Source: CAD feature listing. Evaluate the final solid. Frame: model axes, mm. Coordinates: 2 decimals unless noted, no trailing zeros. Loops run counter-clockwise (first coordinate to the right, second up) from the corner with the lowest first, then second, coordinate; pieces in that order, holes last. Notation, with made-up numbers: (34, 18.5) -> (63, 18.5) arc R21 ccw to (63, 37.5) -> close; hole circle Ø7 at (43, 70.5). An arc over 180 degrees is marked (long way). Answer as a JSON object with one key per item and string values. Group by question number.
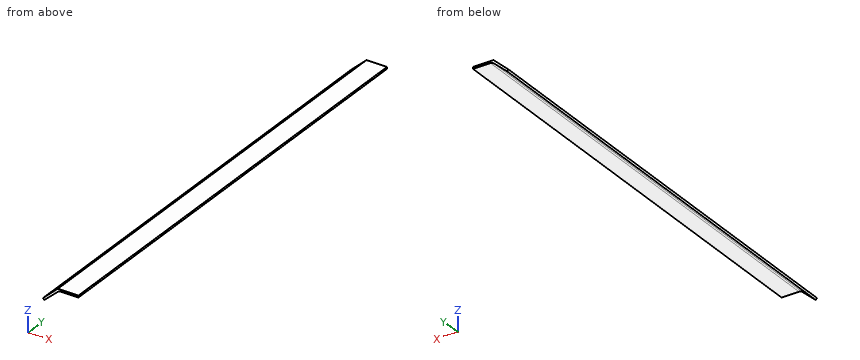
from build123d import *

# Parameters (mm, degrees)
EXTRUDE_START   = 40
EXTRUDE_1_DEPTH = 468.213673317


with BuildPart() as part:
    # Эскиз1 → Вытянуть1 (new body)
    with BuildSketch(Plane(origin=(0, 0, 0), x_dir=(1, 0, 0), z_dir=(0, 1, 0)).offset(EXTRUDE_START)):
        with BuildLine():
            Line((-18.902286518, 12.381871272), (-17.552748119, 13.857928896))
            Line((-17.552748119, 13.857928896), (-3.97119008, 1.754112541))
            ThreePointArc((-3.97119008, 1.754112541), (-2.424474286, 0.81441735), (-0.644564969, 0.48688167))
            Line((-0.644564969, 0.48688167), (17.122829042, 0.48688167))
            Line((17.122829042, 0.48688167), (17.122829042, -1.51311833))
            Line((17.122829042, -1.51311833), (-3.70464164, -1.51311833))
            Line((-3.70464164, -1.51311833), (-18.902286518, 12.381871272))
        make_face()
    extrude(amount=EXTRUDE_1_DEPTH)


solid = part.part
1. Section query B-B on x = 11.5. Return loops of the section in (y, z), then the cut area to 3 significant figures.
2. Section query A-A on y = 181. Return loops of the section in (x, z), then the cut area to 3 significant figures.
3. Section query C-C on z = -7.25. Return loops of the section in (x, y), then the cut area to 3 significant figures.
4. Ray query, L1, parallel to Z at x = 10, y = 412.5; L2, parallel to X at y = 224.5, z = -3; L3, parallel to X at y = 279.5, z = -9.75. Return the intervals inside material, ascending.
5. Pin query (flat end, axial travel): pin 1 Ø3 at (x, y) = (-6.5, 283.5) entering from -Z; pin 2 Ø2 at (y, z) = (163, -3) entering from -X; pin 3 Ø1 at (y, z) = (186.5, -6.5) entering from +X. Return the tip coordinate at first contact, or that it passes through.
Solved:
{
 "1": {"outline": "(40, -0.49) -> (508.21, -0.49) -> (508.21, 1.51) -> (40, 1.51) -> close", "area": "936 mm^2"},
 "2": {"outline": "(-18.9, -12.38) -> (-17.55, -13.86) -> (-3.97, -1.75) arc R5 cw to (-0.64, -0.49) -> (17.12, -0.49) -> (17.12, 1.51) -> (-3.7, 1.51) -> close", "area": "84.2 mm^2"},
 "3": {"outline": "(-13.29, 40) -> (-10.14, 40) -> (-10.14, 508.21) -> (-13.29, 508.21) -> close", "area": "1,480 mm^2"},
 "4": {"L1": "-0.49 to 1.51", "L2": "-8.64 to -5.37", "L3": "-16.02 to -12.94"},
 "5": {"pin 1": "z = -5.34", "pin 2": "x = -9.73", "pin 3": "x = -8.74"}
}
